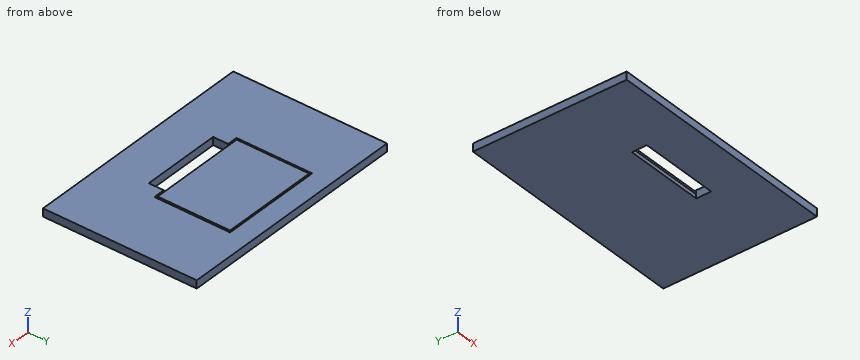
```python
from build123d import *

# Parameters (mm, degrees)
F0_W     = 151.6449451447
F0_H     = 98.8437831402
F1_DEPTH = 5.08
F2_W     = 51.2981526554
F2_H     = 9.6649971419
F3_DEPTH = 25.146
F4_W     = 63.0413852632
F4_H     = 46.5789679438
F5_DEPTH = 2.54


with BuildPart() as f1:
    # F0 (on Top) → F1 (new body)
    with BuildSketch(Plane.XY):
        with Locations((-0.081807375, 6.1048939824)):
            Rectangle(F0_W, F0_H)
    extrude(amount=F1_DEPTH)

    # F2 (on Top) → F3 (cut)
    with BuildSketch(Plane.XY):
        with Locations((0, -10.8838873326)):
            Rectangle(F2_W, F2_H)
    extrude(amount=F3_DEPTH, mode=Mode.SUBTRACT)

    # F4 (on face) → F5 (cut)
    with BuildSketch(Plane.XY.offset(5.08)):
        Polygon((-32.2755798697, 42.5956249237), (-32.2755798697, -6.0513887617), (-25.6490763277, -6.0513887617), (25.6490763277, -6.0513887617), (33.1190824509, -6.0513887617), (33.1190824509, 42.5956249237), align=None)
        with Locations((0.2893041819, 18.2428015396)):
            Rectangle(F4_W, F4_H, mode=Mode.SUBTRACT)
    extrude(amount=-F5_DEPTH, mode=Mode.SUBTRACT)


solid = f1.part
```
Geometry: final body of the model. Coordinates: model frame, mm. Round coordinates to 2 decimals unless told otherwise and drop trailing zeros. Loops run counter-clockwise (first coordinate to the right, second up) from the corner with the lowest first, then second, coordinate; pieces in that order, holes last. Notation, with made-up numbers: (-39, 85.25) -> (-14, 85.25) arc R17 cw to (-14, 110.25) -> close; hole circle Ø2 at (1, 73). An arc over 180 degrees is marked (long way). Write each question's results on one line, items separated by ' | '.
Item 1: Cut plane A-A on z = 4.3. Return the cut outline in (x, y).
Answers below:
outline: (-75.9, -43.32) -> (75.74, -43.32) -> (75.74, 55.53) -> (-75.9, 55.53) -> close; (-31.23, -5.05) -> (31.81, -5.05) -> (31.81, 41.53) -> (-31.23, 41.53) -> close; hole (-32.28, -6.05) -> (-25.65, -6.05) -> (-25.65, -15.72) -> (25.65, -15.72) -> (25.65, -6.05) -> (33.12, -6.05) -> (33.12, 42.6) -> (-32.28, 42.6) -> close
Item 2: Cut plane B-B on x = -6. Return the cut outline in (y, z), and give its area (3 significant figures).
Answers below:
outline: (-43.32, 0) -> (-15.72, 0) -> (-15.72, 5.08) -> (-43.32, 5.08) -> close; (-6.05, 0) -> (55.53, 0) -> (55.53, 5.08) -> (42.6, 5.08) -> (42.6, 2.54) -> (41.53, 2.54) -> (41.53, 5.08) -> (-5.05, 5.08) -> (-5.05, 2.54) -> (-6.05, 2.54) -> close | area: 448 mm²
Item 3: Pin query (flat end, axial travel): pin 1 Ø1 at (x, y) = (-11.5, 37) entering from -Z. Return the tip coordinate at first contact, or that it passes through.
Answers below:
pin 1: stops at z = 0
Item 4: Line query: probe 1 along X at (y, z) = (28.5, 4.5); probe 2 along Y at (x, z) = (0.5, 3); probe 3 along X at (y, z) = (-9, 3.7). Output: solid intervals per line, ascending. Write a range as [from, to].
Answers below:
probe 1: x = [-75.9, -32.28], [-31.23, 31.81], [33.12, 75.74] | probe 2: y = [-43.32, -15.72], [-5.05, 41.53], [42.6, 55.53] | probe 3: x = [-75.9, -25.65], [25.65, 75.74]
